The listing builds one solid part. Answer for the finished solid, in the listing's coordinates (mm). A direction names the side the tool comes from. Give positions to 0.01 mm unless a question says otherwise; leave off trailing zeros. Order: outer loops, then holes, each group sorted by start corner. A loop starts at its lowest first (then second) coordinate and runs counter-clockwise, first axis right, second up.
```python
from build123d import *

# Parameters (mm, degrees)
F0_R     = 3
F1_DEPTH = 1
F2_W     = 5
F2_H     = 2
F3_DEPTH = 7
F4_R     = 2.49999
F5_R     = 1
F6_DEPTH = 4


# Not quite as in the source:
# - a fillet or chamfer is up to 0.001 mm smaller than in the source, because OpenCascade refuses the exact size


with BuildPart() as f1:
    # F0 (on Top) → F1 (new body)
    with BuildSketch(Plane.XY):
        Circle(F0_R)
    extrude(amount=F1_DEPTH)

    # F2 (on face) → F3 (join)
    with BuildSketch(Plane.XY.offset(1)):
        Rectangle(F2_W, F2_H)
    extrude(amount=F3_DEPTH)

    # F4 (radius 2.5 in the source; OpenCascade refuses exactly that, so slightly less here)
    f4_edges = [f1.edges().sort_by_distance(p)[0] for p in [
        (-2.5, 0, 8),
        (2.5, 0, 8),
    ]]
    fillet(f4_edges, radius=F4_R)

    # F5 (on face) → F6 (cut)
    with BuildSketch(Plane.XZ.offset(1)):
        with Locations((0, 5.5)):
            Circle(F5_R)
    extrude(amount=-F6_DEPTH, mode=Mode.SUBTRACT)


solid = f1.part
```
1) For a pull along X with two mould halves and no side action, classify faces 6 (the cylindrical face through (-0.13, -0.01, 6.49)), 7 (the flat face through (0, -1.3, 1)), 8 (the flat face through (2.5, 0, 3)) as +X half, -X half, draft (parallel to the pull), parting line (faces both ways), or undercut.
Geometry says:
face 6: undercut
face 7: draft
face 8: +X half
2) Find section B-B (x = -1.7). Write down the section's boundary in (y, z).
Geometry says:
outline: (-2.47, 0) - (2.47, 0) - (2.47, 1) - (1, 1) - (1, 7.33) - (-1, 7.33) - (-1, 1) - (-2.47, 1) - close
3) Given P1, Ø3, axis at y = -1.5, z = 6, coming from the -X side; P2, Ø1.6, axis at y = 0, z = 3, coming from the +X side; P3, Ø2.5, axis at x = -1, z = 4.5, coming from the -Y side; P4, Ø1.8, axis at x = 0, z = 5.5, coming from the +Y side, each flat-ended and moving along its own axis, determine where each tip first touches the part or whether it passes through.
Geometry says:
P1: stops at x = -2.5
P2: stops at x = 2.5
P3: stops at y = -1
P4: passes through
4) Find section D-D (y = -2.35). Write down the section's boundary in (x, z), then the cut area to 3 significant figures.
Geometry says:
outline: (-1.86, 0) - (1.86, 0) - (1.86, 1) - (-1.86, 1) - close
area: 3.73 mm2
5) Straight lines are drawn through the part: probe 1 along Z at (x, y) = (0, 0.5); probe 2 along Y at (x, z) = (2.45, 4.25); probe 3 along Z at (x, y) = (1.1, -2.65). For each, find the intervals that lie inside material, in ascending order.
Geometry says:
probe 1: z = 0 to 4.5, 6.5 to 8
probe 2: y = -1 to 1
probe 3: z = 0 to 1
6) A tool of negligible diameter and unlimited length cuts with its end or side. For faces 1 (the flat face through (0, 1, 4)), 2 (the flat face through (0, -1, 4)), 3 (the flat face through (-2.5, 0, 3)), 4 (the cylindrical face through (-3, 0.1, 0.5)), 5 (the cylindrical face through (2, 0, 7)), from which of +Z, -Z, +X, -X, +Y, -Y can it reach the whole face along a straight path? Write none if from no direction.
Geometry says:
face 1: +Z, +X, -X, +Y
face 2: +Z, +X, -X, -Y
face 3: +Z, -X, +Y, -Y
face 4: +Z, -Z
face 5: +Z, +X, +Y, -Y
7) Find section C-C (z = 7). Write down the section's boundary in (x, y), then the cut area to 3 significant figures.
Geometry says:
outline: (-2, -1) - (2, -1) - (2, 1) - (-2, 1) - close
area: 8.00 mm2
